Here's how the part is built. I have some questions about the finished solid (model axes, mm). A direction names the side the tool comes from. Give positions to 0.01 mm unless a question says otherwise; leave off trailing zeros. Loops run counter-clockwise (first coordinate to the right, second up) from the corner with the lowest first, then second, coordinate; pieces in that order, holes last. Notation, with made-up numbers: M 64.5,72 L 93.5,72 A28 ccw 93.5,105 Z; hole C 43,15.25 d11. An arc over 180 degrees is marked long. Write item = value, one per line. Start each with the question number.
```python
from build123d import *

# Parameters (mm, degrees)
F1_DEPTH  = 76.2
F3_DEPTH  = 25.4
F5_DEPTH  = 101.6
F7_DEPTH  = 76.2
F10_DEPTH = 37.338
F12_DEPTH = 37.338
F13_R     = 8.807305
F14_DEPTH = 101.6
F15_R     = 3.664816
F16_DEPTH = 116.84
F18_R     = 1.744402
F19_DEPTH = 225.298
F20_R     = 1.703793
F21_DEPTH = 213.106
F22_R     = 1.272162
F23_DEPTH = 254
F25_W     = 23.404523
F25_H     = 20.684985
F26_DEPTH = 209.804
F27_W     = 23.239702
F27_H     = 21.014627
F28_DEPTH = 223.774
F29_W     = 16.646877
F29_H     = 24.311038
F30_DEPTH = 495.046
F31_W     = 16.317241
F31_H     = 23.486935
F32_DEPTH = 242.062
F33_W     = 17.470982
F33_H     = 23.981396
F34_DEPTH = 243.84
F35_W     = 14.833849
F35_H     = 23.816576
F36_DEPTH = 196.85


with BuildPart() as f1:
    # F0 (on Right) → F1 (new body)
    with BuildSketch(Plane.YZ):
        with BuildLine():
            Line((-33.445477, 0), (0, 0))
            ThreePointArc((0, 0), (1.073615, 2.388963), (0, 4.777925))
            ThreePointArc((0, 4.777925), (-16.903377, 3.653432), (-33.445477, 0))
        make_face()
    extrude(amount=F1_DEPTH)

    # F2 (on Right) → F3 (join)
    with BuildSketch(Plane.YZ):
        with BuildLine():
            Line((-21.430658, 0), (0, 0))
            ThreePointArc((0, 0), (1.05119, 2.362129), (0, 4.724259))
            ThreePointArc((0, 4.724259), (-10.876771, 3.094479), (-21.430658, 0))
        make_face()
    extrude(amount=-F3_DEPTH)

    # F4 (on Right) → F5 (join)
    with BuildSketch(Plane.YZ):
        with BuildLine():
            Line((-21.460172, 0), (0, 0))
            ThreePointArc((0, 0), (1.120071, 2.226999), (0, 4.453998))
            ThreePointArc((0, 4.453998), (-10.919842, 3.14128), (-21.460172, 0))
        make_face()
    extrude(amount=F5_DEPTH)

    # F6 (on Right) → F7 (join)
    with BuildSketch(Plane.YZ):
        with BuildLine():
            Line((-23.889625, 1.37669), (0, 4.777925))
            ThreePointArc((0, 4.777925), (-7.260951, 24.620526), (-23.889625, 37.656531))
            Line((-23.889625, 37.656531), (-23.889625, 1.37669))
        make_face()
    extrude(amount=F7_DEPTH)

    # F9 (on offset) → F10 (cut)
    with BuildSketch(Plane.YZ.offset(78.74)):
        with BuildLine():
            ThreePointArc((-34.90315, 0), (-17.651622, 3.850321), (0, 4.777925))
            ThreePointArc((0, 4.777925), (6.961202, 43.833079), (-31.663876, 52.881103))
            ThreePointArc((-31.663876, 52.881103), (-51.316385, 27.545169), (-34.90315, 0))
        make_face()
    extrude(amount=-F10_DEPTH, mode=Mode.SUBTRACT)

    # F11 (on Right) → F12 (cut)
    with BuildSketch(Plane.YZ):
        with BuildLine():
            ThreePointArc((-34.41726, 0), (-17.405812, 3.881122), (0, 5.101853))
            ThreePointArc((0, 5.101853), (12.801217, 34.08098), (-9.798795, 56.282341))
            ThreePointArc((-9.798795, 56.282341), (-55.391799, 42.699829), (-34.41726, 0))
        make_face()
    extrude(amount=F12_DEPTH, mode=Mode.SUBTRACT)

    # F13 (on offset) → F14 (cut)
    with BuildSketch(Plane.YZ.offset(78.74)):
        with Locations((-14.009847, 15.791448)):
            Circle(F13_R)
    extrude(amount=-F14_DEPTH, mode=Mode.SUBTRACT)

    # F15 (on offset) → F16 (cut)
    with BuildSketch(Plane.YZ.offset(78.74)):
        with Locations((-18.544829, 29.396387)):
            Circle(F15_R)
    extrude(amount=-F16_DEPTH, mode=Mode.SUBTRACT)

    # F18 (on offset) → F19 (cut)
    with BuildSketch(Plane.YZ.offset(159.258)):
        with Locations((-1.862581, 2.186508)):
            Circle(F18_R)
    extrude(amount=-F19_DEPTH, mode=Mode.SUBTRACT)

    # F20 (on offset) → F21 (cut)
    with BuildSketch(Plane.YZ.offset(159.258)):
        with Locations((-5.93065, 1.889733)):
            Circle(F20_R)
    extrude(amount=-F21_DEPTH, mode=Mode.SUBTRACT)

    # F22 (on offset) → F23 (cut)
    with BuildSketch(Plane.YZ.offset(159.258)):
        with Locations((-9.853734, 1.698055)):
            Circle(F22_R)
    extrude(amount=-F23_DEPTH, mode=Mode.SUBTRACT)

    # F25 (on offset) → F26 (cut)
    with BuildSketch(Plane.XY.offset(-90.932)):
        with Locations((-13.10903, -10.342492)):
            Rectangle(F25_W, F25_H)
    extrude(amount=F26_DEPTH, mode=Mode.SUBTRACT)

    # F27 (on offset) → F28 (cut)
    with BuildSketch(Plane.XY.offset(-90.932)):
        with Locations((89.32697, -10.507313)):
            Rectangle(F27_W, F27_H)
    extrude(amount=F28_DEPTH, mode=Mode.SUBTRACT)

    # F29 (on offset) → F30 (cut)
    with BuildSketch(Plane.XY.offset(-90.932)):
        with Locations((66.746547, -12.155519)):
            Rectangle(F29_W, F29_H)
    extrude(amount=F30_DEPTH, mode=Mode.SUBTRACT)

    # F31 (on offset) → F32 (cut)
    with BuildSketch(Plane.XY.offset(-90.932)):
        with Locations((9.718621, -11.743467)):
            Rectangle(F31_W, F31_H)
    extrude(amount=F32_DEPTH, mode=Mode.SUBTRACT)

    # F33 (on offset) → F34 (cut)
    with BuildSketch(Plane.XY.offset(-90.932)):
        with Locations((27.766475, -11.990698)):
            Rectangle(F33_W, F33_H)
    extrude(amount=F34_DEPTH, mode=Mode.SUBTRACT)

    # F35 (on offset) → F36 (cut)
    with BuildSketch(Plane.XY.offset(-90.932)):
        with Locations((49.687614, -11.908288)):
            Rectangle(F35_W, F35_H)
    extrude(amount=F36_DEPTH, mode=Mode.SUBTRACT)


solid = f1.part
```
Q1. Will these pins go through, and if not, where does the flat tip stop? pin 1 (1.5 mm diameter, centred on x = 17.5, y = -28, fed in from +Z); pin 2 (1.5 mm diameter, centred on y = -15, z = 3.5, fed in from -X); pin 3 (19 mm diameter, centred on y = -8.5, z = 25.5, fed in from -X).
Q2. If I drill on line 1 along X through (y, z) = (-16.5, 2); line 2 along Z through (x, y) = (57.5, -6); line 3 along X through (y, z) = (-21.5, 25), over which ranges is the centre line in solid material (lowest first)?
Q3. On a 3-axis mill with a long thin cutter (end or side, diameter ignored), from which of +Z, -Z, +X, -X, +Y, -Y can I reach the whole of each face in a straight line? I mean faces 5 (the flat face through (10, 0, 2)), 6 (the cylindrical face through (39.43, -7.28, 0.85)). Say none if no direction works.
Q4. If we section it at A-A, the plane x = 54: List the corners of the cut face in (y, z) for me, then the cut area to 3 significant figures.
Q5. We'd pull the mould along Z, two halves only. Please class faces 1 (the cylindrical face through (36.91, -12.19, 4.53)), 2 (the flat face through (-25.4, -8.6, 2.4)), 3 (the cylindrical face through (-12.52, 1.05, 2.32)), 4 (the cylindrical face through (57.77, -7.28, 0.85)): pulls with the +Z half, pulls with the -Z half, needs draft (parallel to the pull), parting line crosses it, or undercut.
Q6. If we section it at B-B, the plane z = 19: List the corners of the cut face in (x, y) for me, then the cut area to 3 significant figures.
Q7. If we section it at C-C, the plane y = -19.5: State how many separate pieces and enclosed holes the cut face has, then the cut area to 3 significant figures.
Q8. If we section it at D-D, the plane x = -8.5: List the corners of the cut face in (y, z) for me.
Resolved:
q1.pin_1 = 1.68
q1.pin_2 = 0
q1.pin_3 = 37.34
q2.line_1 = 0 to 1.56, 17.88 to 19.03, 36.5 to 42.27, 57.1 to 58.42, 75.07 to 76.2
q2.line_2 = 0 to 0.19, 3.59 to 4.79
q2.line_3 = 37.34 to 41.4
q3.face_5 = +Z, -Z
q3.face_6 = +X, -X
q4.outline = M -33.45,0 L -23.82,0 L -23.82,2.82 A105.91 ccw -23.89,2.81 L -23.89,2.43 A112.34 ccw Z; M 0,0 A2.77 ccw 1.02,2.95 A3.19 ccw 0,4.78 Z
q4.area = 16.2 mm²
q5.face_1 = pulls with the +Z half
q5.face_2 = needs draft
q5.face_3 = parting line crosses it
q5.face_4 = undercut
q6.outline = M 37.34,-23.89 L 41.4,-23.89 L 41.4,-22.21 L 37.34,-22.21 Z; M 37.34,-5.81 L 41.4,-5.81 L 41.4,-3.87 L 37.34,-3.87 Z
q6.area = 14.7 mm²
q7.separate_pieces = 9
q7.enclosed_holes = 0
q7.area = 87.1 mm²
q8.outline = M -21.43,0 L -20.68,0 L -20.68,0.27 A80.65 ccw Z; M 0,0 A3.18 ccw 0,4.72 Z
